Design review of the part built by this model. Coordinates are the model's own, in mm. A direction names the side the tool comes from. Coordinates: 2 decimals unless noted, no trailing zeros. Write each loop counter-clockwise with the first axis right and the second up, starting at its lowest first coordinate (ties: lowest second). Pieces come first, ordered by that corner, then holes. Notation, with made-up numbers: M 14.5,42.5 L 31.5,42.5 A5 cw 31.5,50.5 Z; hole C 85,24 d9. An arc over 180 degrees is marked long. Write item = value, one per line.
```python
from build123d import *

# Parameters (mm, degrees)
SKETCH1_R           = 5.8
BOSS_EXTRUDE1_DEPTH = 23
BOSS_EXTRUDE2_DEPTH = 1.25
SKETCH4_R           = 1.3
CUT_EXTRUDE1_DEPTH  = 36.0000001


with BuildPart() as part:
    # Sketch1 → Boss-Extrude1 (new body)
    with BuildSketch(Plane.XY):
        Circle(SKETCH1_R)
    extrude(amount=BOSS_EXTRUDE1_DEPTH)

    # Sketch2 → Boss-Extrude2 (add, symmetric)
    with BuildSketch(Plane(origin=(0, 0, 0), x_dir=(1, 0, 0), z_dir=(0, 1, 0))):
        with BuildLine():
            Line((0, 0), (37, 0))
            ThreePointArc((37, 0), (34.071067812, -7.071067812), (27, -10))
            Line((27, -10), (15.101535324, -10))
            ThreePointArc((15.101535324, -10), (8.030467512, -12.928932188), (5.101535324, -20))
            Line((5.101535324, -20), (0, -20))
            Line((0, -20), (0, 0))
        make_face()
    extrude(amount=BOSS_EXTRUDE2_DEPTH, both=True)

    # Sketch3 → Revolve1 (revolve)
    with BuildSketch(Plane(origin=(0, 0, 0), x_dir=(1, 0, 0), z_dir=(0, 1, 0))):
        with BuildLine():
            Line((0, -23), (-5.8, -23))
            ThreePointArc((-5.8, -23), (-5.536156171, -26.687563559), (-4.75, -30.3))
            Line((-4.75, -30.3), (-3.95, -30.3))
            Line((-3.95, -30.3), (-3.95, -35))
            Line((-3.95, -35), (0, -35))
            Line((0, -35), (0, -23))
        make_face()
    revolve(axis=Axis((0, 0, 1000), (0, 0, -1)))

    # Sketch4 → Cut-Extrude1 (cut, through all)
    with BuildSketch(Plane.XY.offset(35)):
        Circle(SKETCH4_R)
    extrude(amount=-CUT_EXTRUDE1_DEPTH, mode=Mode.SUBTRACT)


solid = part.part
```
Q1. For P1, Ø1.5, axis at y = 3, z = 13, coming from the +X side; P2, Ø12, axis at x = 28, z = 11.5, coming from the -Y side; P3, Ø2, axis at x = 32.5, y = 3, coming from the -Z side; P4, Ø5, axis at x = 21, z = 7, coming from the +Y side, all flat-tipped, find the tip position at first contact; note any pin that passes through.
Check result:
P1 = 5.35
P2 = -1.25
P3 = through
P4 = 1.25
Q2. The part is to be moulded in two halves that separate along X. For faces 1 (the cylindrical face through (-0.17, 1.29, 17.74)), 2 (the cylindrical face through (9.39, 0.02, 11.79)), 3 (the cylindrical face through (3.135, -2.404, 32.683)), say which applies: +X half, -X half, draft (parallel to the pull), parting line (faces both ways), or undercut.
Check result:
face_1 = undercut
face_2 = +X half
face_3 = parting line
Q3. Machinability: for faces 4 (the flat face through (22, -1.25, 5)), 5 (the flat face through (21, 0, 10)), 6 (the flat face through (4, 1, 30.3)), which of the approach directions +Z, -Z, +X, -X, +Y, -Y give a long, thin tool a straight path to every point of the face, cutting with its end or side? Answer none if there is none.
Check result:
face_4 = +Z, -Z, +X, -Y
face_5 = +Z, +X, +Y, -Y
face_6 = +Z
Q4. Consider section A-A, the plane z = 31.5. State the section outline as (x, y) points, and give its area (3 significant figures).
Check result:
outline = C 0,0 d7.9; hole C 0,0 d2.6
area = 43.7 mm²
Q5. Consider section B-B, the plane x = 17. State the section outline as (y, z) points.
Check result:
outline = M -1.25,0 L 1.25,0 L 1.25,10 L -1.25,10 Z
Q6. Wall thickness on line 1 (Y direction, x = 0, z = 20); line 2 (Z direction, x = 2.5, y = 3.5); line 3 (X direction, y = 0.75, z = 25): over which ranges is each line inside the solid? List them lowest first.
Check result:
line_1 = -5.8 to -1.3, 1.3 to 5.8
line_2 = 0 to 30.3
line_3 = -5.67 to -1.06, 1.06 to 5.67
Q7. Consider section C-C, the plane x = 32.5. State the section outline as (y, z) points.
Check result:
outline = M -1.25,0 L 1.25,0 L 1.25,8.35 L -1.25,8.35 Z
